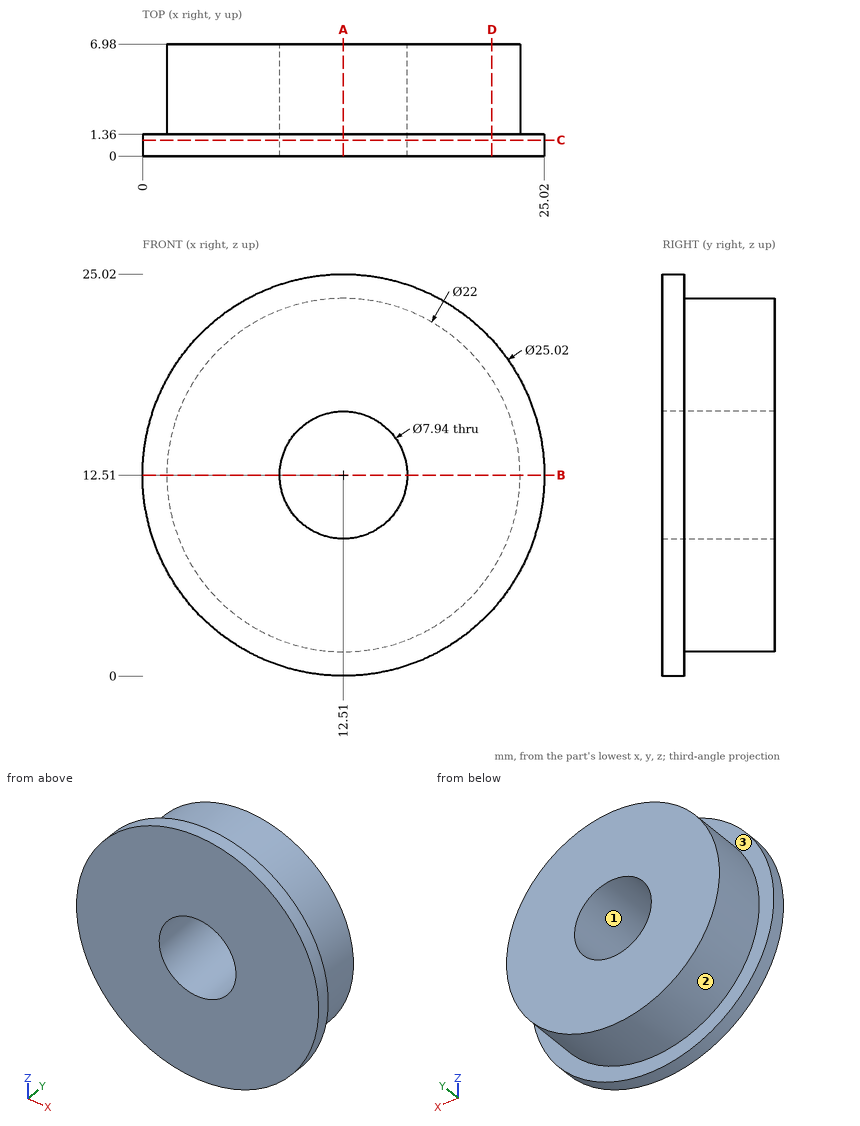
The drawing under review shows one solid part. Ordinate dimensions are in mm from its lowest x, y, z. Round coordinates to 2 decimals unless told otherwise and drop trailing zeros. Write each loop counter-clockwise with the first axis right and the second up, starting at its lowest first coordinate (ties: lowest second). Pieces come first, ordered by that corner, then holes. Notation, with made-up numbers: (-38, 82) -> (-12, 82) arc R19 ccw to (-12, 106) -> close; hole circle Ø3 at (9, -27). An arc over 180 degrees is marked (long way). Put each result on its own line as item: value.
Q1. Consider section B-B on z = 12.51. State the section outline as (x, y) points.
Determined:
outline: (0, 0) -> (8.54, 0) -> (8.54, 6.98) -> (1.51, 6.98) -> (1.51, 1.36) -> (0, 1.36) -> close; (16.48, 0) -> (25.02, 0) -> (25.02, 1.36) -> (23.51, 1.36) -> (23.51, 6.98) -> (16.48, 6.98) -> close
Q2. Consider section A-A on x = 12.51. State the section outline as (y, z) points.
Determined:
outline: (0, 0) -> (1.36, 0) -> (1.36, 1.51) -> (6.98, 1.51) -> (6.98, 8.54) -> (0, 8.54) -> close; (0, 16.48) -> (6.98, 16.48) -> (6.98, 23.51) -> (1.36, 23.51) -> (1.36, 25.02) -> (0, 25.02) -> close
Q3. Clearance check with flat-ended pins moving along their axes: pin 1 Ø2 at (y, z) = (6, 18.5) entering from -X; pin 2 Ø5 at (x, z) = (21, 15) entering from -Y; pin 3 Ø3 at (x, y) = (4.5, 5.5) entering from +Z; pin 4 Ø2 at (y, z) = (1, 14.5) entering from +X. State where each tip first meets the part, or that it passes through.
Determined:
pin 1: stops at x = 2.71
pin 2: stops at y = 0
pin 3: stops at z = 21.38
pin 4: stops at x = 24.98
Q4. To check wall thickness, follow L1, parallel to Z at x = 9.5, y = 5; L2, parallel to X at y = 2.5, z = 11.25; L3, parallel to X at y = 4, z = 13.25. State the ranges of each line that lie inside material, in increasing order. Write a range as [from, to].
Determined:
L1: z = [1.93, 9.92], [15.1, 23.09]
L2: x = [1.58, 8.75], [16.27, 23.44]
L3: x = [1.53, 8.61], [16.41, 23.49]
Q5. Consider section D-D on x = 21.75. State the section outline as (y, z) points, and give its area (3 significant figures).
Determined:
outline: (0, 4.08) -> (1.36, 4.08) -> (1.36, 6.54) -> (6.98, 6.54) -> (6.98, 18.48) -> (1.36, 18.48) -> (1.36, 20.94) -> (0, 20.94) -> close
area: 90.0 mm^2
Q6. Consider section C-C on y = 1. State the section outline as (x, z) points.
Determined:
outline: circle Ø25.02 at (12.51, 12.51); hole circle Ø7.94 at (12.51, 12.51)
Q7. The part is to be moulded in two halves that separate along X. For the marked faces 1, 2 and 3, say which applies: released by +X, released by -X, zero draft, split by the parting line, or undercut.
Determined:
face 1: undercut
face 2: split by the parting line
face 3: zero draft
